from build123d import *

# Parameters (mm, degrees)
SKETCH1_R           = 19.5
SKETCH1_R_2         = 15
BOSS_EXTRUDE1_DEPTH = 270
SKETCH3_W           = 2.5
SKETCH3_H           = 30
BOSS_EXTRUDE2_DEPTH = 6


with BuildPart() as part:
    # Sketch1 → Boss-Extrude1 (new body)
    with BuildSketch(Plane(origin=(0, 0, 0), x_dir=(1, 0, 0), z_dir=(0, 1, 0))):
        Circle(SKETCH1_R)
        Circle(SKETCH1_R_2, mode=Mode.SUBTRACT)
    extrude(amount=BOSS_EXTRUDE1_DEPTH)

    # Sketch3 → Boss-Extrude2 (add)
    with BuildSketch(Plane.XY.offset(22.5)):
        with Locations((0, 156.116903923)):
            Rectangle(SKETCH3_W, SKETCH3_H)
    extrude(amount=-BOSS_EXTRUDE2_DEPTH)


solid = part.part
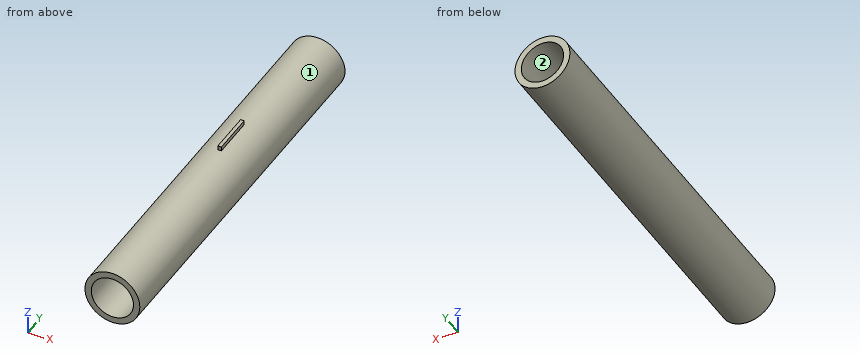
Check sheet for the modelled part. Datum: model origin and axes. Units: mm. Face numbers are marked on the shaded views. Round coordinates to 2 decimals unless told otherwise and drop trailing zeros. Order: outer loops, then holes, each group sorted by start corner. A loop starts at its lowest first (then second) coordinate and runs counter-clockwise, first axis right, second up. Notation, with made-up numbers: M 28,66 L 33,66 A12 ccw 33,79 Z; hole C 70.5,-31.75 d6. An arc over 180 degrees is marked long. One line per item, written item: value. Start each with the question number.
1. Section check D-D on y = 191. Enter the section's corners in (x, z), and give its area (3 significant figures).
2. Section check A-A on z = 0. Enter the section's corners in (x, y).
3. Scan lines: line 1 along X through (y, z) = (185, 0); line 2 along X through (y, z) = (78, 10). Record each from-to range of solid material in increasing order.
4. Section check C-C on y = 154. Enter the section's corners in (x, z), and give its area (3 significant figures).
5. Section check B-B on x = 3.5. Enter the section's corners in (y, z), and give its area (3 significant figures).
6. Release check for a two-part mould opening along Z. For the marked faces 1 and 2 record: released by +Z, released by -Z, zero draft, split by the parting line, or undercut.
7. Gauge pin test, flat ends, axial feed: P1, Ø1, axis at y = 211.5, z = -3, coming from the -X side; P2, Ø2.5, axis at y = 155, z = 21, coming from the -X side; P3, Ø8, axis at x = 2, y = 124, coming from the -Z side; P4, Ø1, axis at x = 3, z = -13.5, coming from the +Y side. Record the tip position at first contact, or that the pin passes through.
Results found:
1. outline: C 0,0 d39; hole C 0,0 d30
1. area: 488 mm^2
2. outline: M -19.5,0 L -15,0 L -15,270 L -19.5,270 Z; M 15,0 L 19.5,0 L 19.5,270 L 15,270 Z
3. line 1: -19.5 to -15, 15 to 19.5
3. line 2: -16.74 to -11.18, 11.18 to 16.74
4. outline: M -1.25,19.46 A19.5 ccw long 1.25,19.46 L 1.25,22.5 L -1.25,22.5 Z; hole C 0,0 d30
4. area: 495 mm^2
5. outline: M 0,-19.18 L 270,-19.18 L 270,-14.59 L 0,-14.59 Z; M 0,14.59 L 270,14.59 L 270,19.18 L 0,19.18 Z
5. area: 2,480 mm^2
6. face 1: split by the parting line
6. face 2: undercut
7. P1: x = -19.34
7. P2: x = -1.25
7. P3: z = -19.5
7. P4: through
